Could you check a few things on this model? Use its own coordinates, in mm. Face numbers are marked on the shaded views. A direction names the side the tool comes from. Round coordinates to 2 decimals unless told otherwise and drop trailing zeros. Loops run counter-clockwise (first coordinate to the right, second up) from the corner with the lowest first, then second, coordinate; pieces in that order, holes last. Notation, with made-up numbers: (-21.75, 39) -> (-17.75, 39) arc R28 ccw to (-17.75, 63) -> close; hole circle Ø1 at (1, -18.5). An arc over 180 degrees is marked (long way). One line per item, written item: value.
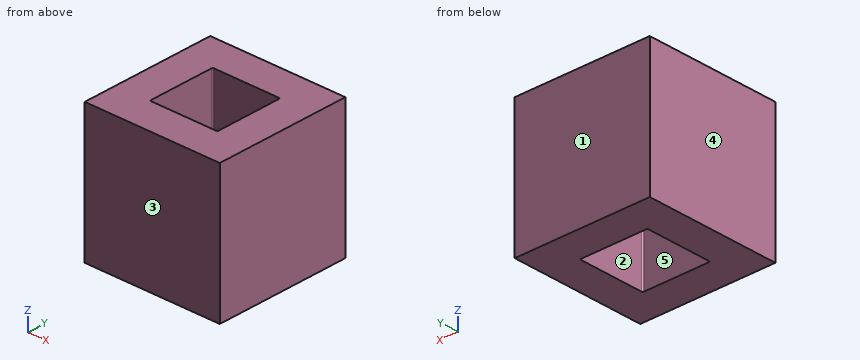
from build123d import *

# Parameters (mm, degrees)
F0_W     = 101.6
F0_H     = 101.6
F1_DEPTH = 50.8
F2_W     = 50.8
F2_H     = 50.8
F3_DEPTH = 50.8
F4_R     = 1.016


with BuildPart() as f1:
    # F0 (on Front) → F1 (new body, symmetric)
    with BuildSketch(Plane.XZ):
        Rectangle(F0_W, F0_H)
    extrude(amount=F1_DEPTH, both=True)

    # F2 (on Top) → F3 (cut, symmetric)
    with BuildSketch(Plane.XY):
        Rectangle(F2_W, F2_H)
    extrude(amount=F3_DEPTH, both=True, mode=Mode.SUBTRACT)

    # F4
    f4_edges = [f1.edges().sort_by_distance(p)[0] for p in [
        (-25.4, -25.4, 0),
        (-25.4, 25.4, 0),
        (25.4, 25.4, 0),
        (25.4, -25.4, 0),
    ]]
    fillet(f4_edges, radius=F4_R)


solid = f1.part
(1) For the marked faces 1 and 2, which set-ups out of +Z, -Z, +X, -X, +Y, -Y let a thin tool reach every point of the face, with its end or its side?
Recorded:
face 1: +Z, -Z, +X, -X, +Y
face 2: +Z, -Z
(2) Thinking about a two-plate mould opening in X: for the marked faces 3, 4 and 5, which applies, released by +X, released by -X, zero draft, split by the parting line, or undercut?
Recorded:
face 3: zero draft
face 4: released by -X
face 5: undercut
(3) If we section it at A-A, the plane y = -5: Please give me the cut outline in (x, z).
Recorded:
outline: (-50.8, -50.8) -> (-25.4, -50.8) -> (-25.4, 50.8) -> (-50.8, 50.8) -> close; (25.4, -50.8) -> (50.8, -50.8) -> (50.8, 50.8) -> (25.4, 50.8) -> close
(4) If we section it at C-C, the plane z = -39: Please give me the cut outline in (x, y), then the cut area to 3 significant figures.
Recorded:
outline: (-50.8, -50.8) -> (50.8, -50.8) -> (50.8, 50.8) -> (-50.8, 50.8) -> close; hole (-25.4, -24.38) arc R1.02 ccw to (-24.38, -25.4) -> (24.38, -25.4) arc R1.02 ccw to (25.4, -24.38) -> (25.4, 24.38) arc R1.02 ccw to (24.38, 25.4) -> (-24.38, 25.4) arc R1.02 ccw to (-25.4, 24.38) -> close
area: 7,740 mm²
(5) If I drill on L1, parallel to Y at x = -9, z = 33.5, over which ranges is the centre line in solid material (lowest first)?
Recorded:
L1: -50.8 to -25.4, 25.4 to 50.8
